from build123d import *

# Parameters (mm, degrees)
SKETCH1_R           = 1.975
SKETCH1_R_2         = 1.554999938
BOSS_EXTRUDE1_DEPTH = 4.5


with BuildPart() as part:
    # Sketch1 → Boss-Extrude1 (new body)
    with BuildSketch(Plane(origin=(0, 0, 0), x_dir=(1, 0, 0), z_dir=(0, 1, 0))):
        with BuildLine():
            Line((-16.144899663, 8.454003274), (10.877745108, 8.454003274))
            ThreePointArc((10.877745108, 8.454003274), (16.961539544, 3.139522495), (12.51277209, -3.603231306))
            ThreePointArc((12.51277209, -3.603231306), (10.56783567, -4.367093581), (8.824099884, -5.518461795))
            add(Edge.make_bspline(
                [(8.824099884, -5.518461795), (4.932532744, -8.718832913), (-4.696045283, -16.58586855), (-31.489086781, -46.943790059), (-12.894682963, -87.326546642), (-17.517744483, -112.138995974)],
                knots=[0.023478108, 0.023478108, 0.023478108, 0.023478108, 0.154944007, 0.330832674, 1, 1, 1, 1], degree=3))
            ThreePointArc((-17.517744483, -112.138995974), (-24.835663445, -118.119615453), (-29.239494185, -109.757437382))
            add(Edge.make_bspline(
                [(-32.217521916, -3.987452131), (-42.206514906, -27.827820505), (-29.561370115, -63.982250345), (-27.390169054, -99.665041987), (-29.239494185, -109.757437382)],
                knots=[0, 0, 0, 0, 0.696305279, 0.977824201, 0.977824201, 0.977824201, 0.977824201], degree=3))
            Line((-32.217521916, -3.987452131), (-16.144899663, 8.454003274))
        make_face()
        with Locations(Location((-23.620555115, -4.478995902, 0), (0, 0, 270))):
            Circle(SKETCH1_R, mode=Mode.SUBTRACT)
        with Locations(Location((-23.620555115, -112.138995974, 0), (0, 0, 270))):
            Circle(SKETCH1_R_2, mode=Mode.SUBTRACT)
        with Locations(Location((-23.620555115, -104.378996, 0), (0, 0, 270))):
            Circle(SKETCH1_R_2, mode=Mode.SUBTRACT)
    extrude(amount=BOSS_EXTRUDE1_DEPTH)


solid = part.part
Model file for the job. Use its own axes, mm. Give positions to 0.01 mm unless a question says otherwise; leave off trailing zeros. Return JSON: item names as keys, results as strings.
1) Cut at A-A, the plane y = 0.8. Count the separate pieces of the cut face and the enclosed holes in it, plus the area to 3 significant figures.
Geometry says:
{"separate pieces": "1", "enclosed holes": "3", "area": "2,430 mm²"}
2) Probe line 1 (Z direction, x = -23.5, y = 1.1); line 2 (Z direction, x = -22, y = 0.2); line 3 (X direction, y = 4.15, z = 105.5). List the from-to ranges inside material, lowest first. Write a range as from..to.
Geometry says:
{"line 1": "-2.76..2.51, 6.45..102.83, 105.93..110.59, 113.69..118.24", "line 2": "-3.92..3.35, 5.61..118.02", "line 3": "-28.6..-24.7, -22.54..-16.72"}
3) Flat gauge pins, fed straight in: P1, Ø3.5, axis at x = -23.62, z = 112.14, coming from the +Y side; P2, Ø1, axis at y = 3.5, z = 36.5, coming from the -X side; P3, Ø1, axis at x = -18.5, y = 2.5, coming from the +Z side. Where does each tip first touch, or does it go through?
Geometry says:
{"P1": "y = 4.5", "P2": "x = -36.47", "P3": "z = 116.13"}
4) Pull direction X, two halves, no side cores. Call faces 1 (the cylindrical face through (-24.687, 2.218, 118.148)), 2 (the flat face through (-19, 0, 36)), 3 (the cylindrical face through (-22.08, 2.22, 104.18)): pulls with the +X half, pulls with the -X half, needs draft (parallel to the pull), parting line crosses it, or undercut.
Geometry says:
{"face 1": "parting line crosses it", "face 2": "needs draft", "face 3": "undercut"}
